```python
from build123d import *

# Parameters (mm, degrees)
P_IDAT_VYSUNUT_M2_DEPTH  = 105
SKICA3_W                 = 30
SKICA3_H                 = 12
ODEBRAT_VYSUNUT_M1_DEPTH = 102
SKICA5_W                 = 6
SKICA5_H                 = 2
ODEBRAT_VYSUNUT_M3_DEPTH = 15
ODEBRAT_VYSUNUT_M6_DEPTH = 102
SKICA12_W                = 41
SKICA12_H                = 20
ODEBRAT_VYSUNUT_M8_DEPTH = 2
SKICA13_W                = 13.4
SKICA13_H                = 5.8
ODEBRAT_VYSUNUT_M9_DEPTH = 10
ZAOBLIT1_R               = 2
ZAOBLIT2_R               = 2
ZKOSEN_2_SIZE            = 3


# Some blends are built 0.0001 mm under size
with BuildPart() as part:
    # Skica2 → Přidat vysunutím2 (new body)
    with BuildSketch(Plane(origin=(0, 0, 0), x_dir=(0, 0, -1), z_dir=(1, 0, 0))):
        Polygon((15.558367755, 10), (-30, 10), (-30, -10), (30, -10), (30, 10), (21.59358807, 10), (23, -2.961048892), (21.5, -2.961048892), (26, -5), (26, -7), (14, -7), (14, -5), (18.5, -2.961048892), (16.964779685, -2.961048892), align=None)
    extrude(amount=P_IDAT_VYSUNUT_M2_DEPTH)

    # Skica3 → Odebrat vysunutím1 (cut)
    with BuildSketch(Plane(origin=(105, 0, 0), x_dir=(0, 0, -1), z_dir=(1, 0, 0))):
        with Locations((-12, -2)):
            Rectangle(SKICA3_W, SKICA3_H)
    extrude(amount=-ODEBRAT_VYSUNUT_M1_DEPTH, mode=Mode.SUBTRACT)

    # Skica5 → Odebrat vysunutím3 (cut)
    with BuildSketch(Plane(origin=(0, 0, -14), x_dir=(-1, 0, 0), z_dir=(0, 0, -1))):
        with Locations((-102, -6)):
            Rectangle(SKICA5_W, SKICA5_H)
    extrude(amount=-ODEBRAT_VYSUNUT_M3_DEPTH, mode=Mode.SUBTRACT)

    # Skica10 → Odebrat vysunutím6 (cut)
    with BuildSketch(Plane(origin=(105, 0, 0), x_dir=(0, 0, -1), z_dir=(1, 0, 0))):
        with BuildLine():
            ThreePointArc((-20.610511889, 7), (-23.90017092, 5.702152702), (-27, 4))
            Line((-27, 4), (3, 4))
            ThreePointArc((3, 4), (-0.09982908, 5.702152702), (-3.389488111, 7))
            Line((-3.389488111, 7), (-20.610511889, 7))
        make_face()
    extrude(amount=-ODEBRAT_VYSUNUT_M6_DEPTH, mode=Mode.SUBTRACT)

    # Skica12 → Odebrat vysunutím8 (cut)
    with BuildSketch(Plane(origin=(105, 0, 0), x_dir=(0, 0, -1), z_dir=(1, 0, 0))):
        with Locations((-9.5, 0)):
            Rectangle(SKICA12_W, SKICA12_H)
    extrude(amount=-ODEBRAT_VYSUNUT_M8_DEPTH, mode=Mode.SUBTRACT)

    # Skica13 → Odebrat vysunutím9 (cut)
    with BuildSketch(Plane.XY.offset(30)):
        with Locations((90.3, -4.1)):
            Rectangle(SKICA13_W, SKICA13_H)
    extrude(amount=-ODEBRAT_VYSUNUT_M9_DEPTH, mode=Mode.SUBTRACT)

    # Zaoblit1
    zaoblit1_edges = [part.edges().sort_by_distance(p)[0] for p in [
        (0, 0, 30),
        (0, 10, 7.220816123),
        (105, 10, -13.279183877),
        (105, 10, -25.796794035),
        (0, 10, -25.796794035),
        (0, 0, -30),
        (52.5, 10, -30),
        (105, 0, -30),
    ]]
    fillet(zaoblit1_edges, radius=ZAOBLIT1_R)

    # Zaoblit2
    # the kernel refuses this fillet: 2 mm, written as the material it takes off along each edge
    with BuildSketch(Plane(origin=(2, 8, 28), x_dir=(0, 0, 1), z_dir=(0, 1, 0))) as zaoblit2_piece_1_section:
        Polygon((0, 0), (ZAOBLIT2_R, 0), (ZAOBLIT2_R, -ZAOBLIT2_R), (0, -ZAOBLIT2_R), align=None)
    zaoblit2_piece_1 = extrude(amount=ZAOBLIT2_R, mode=Mode.PRIVATE)
    zaoblit2_piece_1 = zaoblit2_piece_1 - Plane(origin=(2, 8, 28), x_dir=(0.7071067811865475, 0, -0.7071067811865475), z_dir=(0, 1, 0)) * Sphere(ZAOBLIT2_R, mode=Mode.PRIVATE)
    add(zaoblit2_piece_1, mode=Mode.SUBTRACT)
    with BuildSketch(Plane(origin=(2, 10, 30), x_dir=(0, 0, -1), z_dir=(1, 0, 0))) as zaoblit2_piece_2:
        with BuildLine():
            CenterArc((ZAOBLIT2_R, -ZAOBLIT2_R), ZAOBLIT2_R, 90, 90)
            Line((0, -ZAOBLIT2_R), (0, 0))
            Line((0, 0), (ZAOBLIT2_R, 0))
        make_face()
    extrude(amount=106, mode=Mode.SUBTRACT)

    # Zkosení2
    zkosen_2_edges = [part.edges().sort_by_distance(p)[0] for p in [
        (97, -4.1, 27),
    ]]
    chamfer(zkosen_2_edges, length=ZKOSEN_2_SIZE - 0.0001)  # a hair under: the kernel refuses the full size


solid = part.part
```
Part model, mm, in its own coordinate system. A direction names the side the tool comes from. Give positions to 0.01 mm unless a question says otherwise; leave off trailing zeros. Loops run counter-clockwise (first coordinate to the right, second up) from the corner with the lowest first, then second, coordinate; pieces in that order, holes last. Notation, with made-up numbers: M 29,89.25 L 65,89.25 A10 ccw 65,103.25 Z; hole C -15,75.5 d8. An arc over 180 degrees is marked long. Return JSON: item names as keys, results as strings.
1) Pull direction X, two halves, no side cores. Call faces 4 (the face through (92, -7, 29)), 5 (the face through (51.765, 3.61, -22.287)), 6 (the face through (104.4, -0.87, -29.43)): released by +X, released by -X, zero draft, split by the parting line, or undercut.
Calculated:
{"face 4": "undercut", "face 5": "zero draft", "face 6": "released by +X"}
2) Flat gauge pins, fed straight in: pin 1 Ø1.6 at (x, y) = (104, -8) entering from +Z; pin 2 Ø1.6 at (y, z) = (-6.5, -9.5) entering from +X. Where does each tip first touch, or does it go through?
Calculated:
{"pin 1": "stops at z = -11", "pin 2": "stops at x = 103"}
3) Saw through at C-C, the plane x = 41. List the corners of the cut face in (y, z), then the cut area to 3 significant figures.
Calculated:
{"outline": "M -10,-30 L 8,-30 A2 ccw 10,-28 L 10,-21.59 L -2.96,-23 L -2.96,-21.5 L -5,-26 L -7,-26 L -7,-14 L -5,-14 L -2.96,-18.5 L -2.96,-16.96 L 10,-15.56 L 10,28 A2 ccw 8,30 L -10,30 Z; hole M -8,-3 L 4,-3 A28 ccw 7,3.39 L 7,20.61 A28 ccw 4,27 L -8,27 Z", "area": "648 mm2"}
4) 3-axis set-ups, long thin cutter, end or side, ignore diameter. For faces 1 (the face through (98, -4, 29)), 2 (the face through (54, -8, 12)), 3 (the face through (104, 2, -11)): which of +Z, -Z, +X, -X, +Y, -Y reach the whole face in a straight line?
Calculated:
{"face 1": "none", "face 2": "+X", "face 3": "+Z, +X, +Y, -Y"}
5) Saw through at A-A, the plane z = 16.5. List the corners of the cut face in (x, y).
Calculated:
{"outline": "M 0,-10 L 103,-10 L 103,-8 L 3,-8 L 3,7 L 103,7 L 103,10 L 2,10 A2 ccw 0,8 Z"}
6) Saw through at D-D, the plane z = 24.5. List the corners of the cut face in (x, y), then the cut area to 3 significant figures.
Calculated:
{"outline": "M 0,-10 L 103,-10 L 103,-8 L 3,-8 L 3,5.41 L 103,5.41 L 103,10 L 2,10 A2 ccw 0,8 Z", "area": "718 mm2"}
7) Drill centre lines: line 1 (Y direction, x = 59.5, z = 4); line 2 (Z direction, x = 49, y = -5.5); line 3 (Z direction, x = 70.5, y = 4.25). Where is each one in solid material? Low to high.
Calculated:
{"line 1": "y = -10 to -8, 7 to 10", "line 2": "z = -30 to -26, -14 to -3, 27 to 30", "line 3": "z = -30 to -22.22, -16.18 to -2.6, 26.6 to 30"}
8) Saw through at B-B, the plane y = 5. List the corners of the cut face in (x, z).
Calculated:
{"outline": "M 0,-28 A2 ccw 2,-30 L 103,-30 A2 ccw 105,-28 L 105,-22.14 L 0,-22.14 Z; M 0,-16.1 L 105,-16.1 L 105,-11 L 103,-11 L 103,-1.29 L 3,-1.29 L 3,25.29 L 103,25.29 L 103,30 L 2,30 A2 ccw 0,28 Z"}
